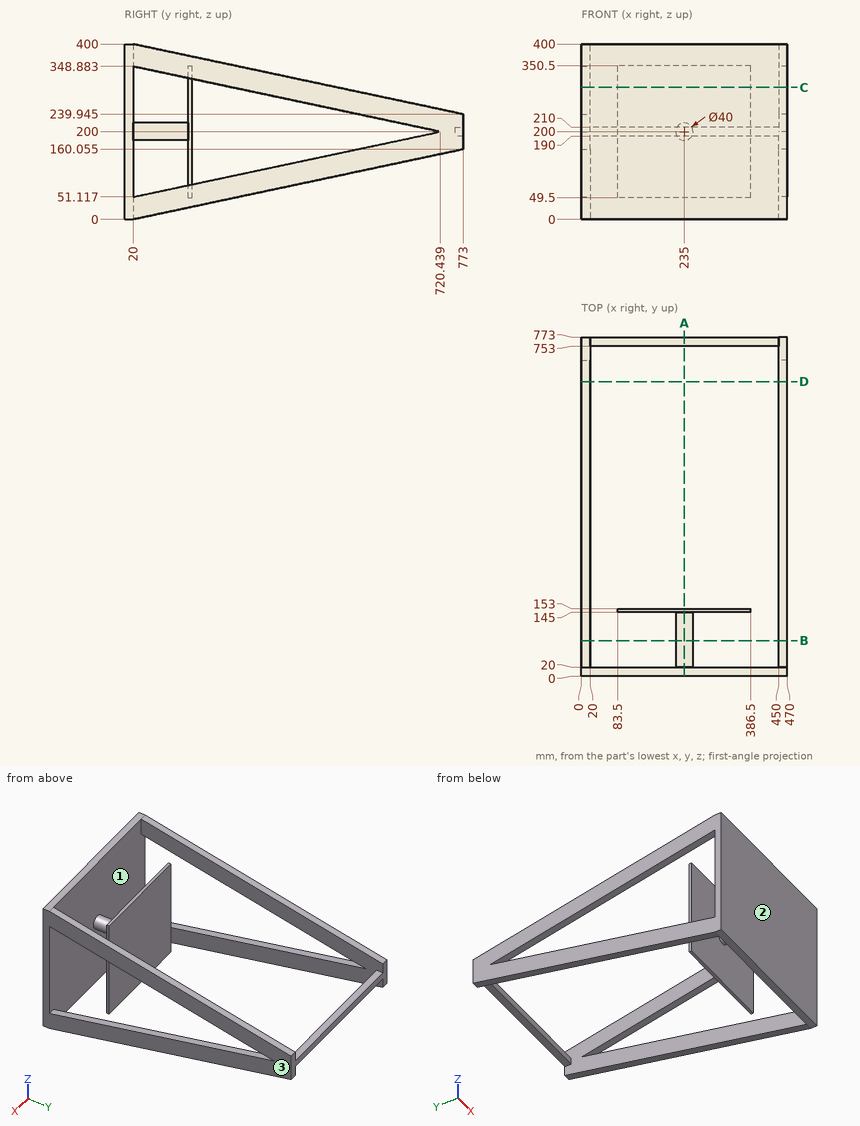
Can you work these out from the drawing? Everything is in mm from the part's minimum corner. Coordinates: 2 decimals unless noted, no trailing zeros. Loops run counter-clockwise (first coordinate to the right, second up) from the corner with the lowest first, then second, coordinate; pieces in that order, holes last. Notation, with made-up numbers: (-38.5, 72.5) - (-10.5, 72.5) arc R25 ccw to (-10.5, 94.5) - close; hole circle Ø9 at (0.5, 22). An arc over 180 degrees is marked (long way). Use a Markdown table: item, result.
Item 1: Will these pins go through, and if not, where does the flat tip stop? pin 1 (10 mm diameter, centred on x = 354.5, y = 146.5, fed in from +Z); pin 2 (22 mm diameter, centred on x = 159.5, y = 762.5, fed in from +Z); pin 3 (4 mm diameter, centred on y = 150, z = 266, fed in from -X).
Numbers:
| item | result |
|---|---|
| pin 1 | stops at z = 350.5 |
| pin 2 | stops at z = 210 |
| pin 3 | stops at x = 83.5 |
Item 2: We'd pull the mould along Y, two halves only. Please class the marked faces 1, 2 and 3: released by +Y, released by -Y, zero draft, split by the parting line, or undercut.
Numbers:
| item | result |
|---|---|
| face 1 | undercut |
| face 2 | released by -Y |
| face 3 | zero draft |
Item 3: I want a section at C-C on z = 301. Please give me the cut outline in (x, y).
Numbers:
| item | result |
|---|---|
| outline | (0, 0) - (470, 0) - (470, 20) - (0, 20) - close; (0, 245.27) - (20, 245.27) - (20, 485.76) - (0, 485.76) - close; (83.5, 145) - (386.5, 145) - (386.5, 153) - (83.5, 153) - close; (450, 245.27) - (470, 245.27) - (470, 485.76) - (450, 485.76) - close |
Item 4: I want a section at B-B on y = 81. Please give me the cut outline in (x, z), and give its area (3 significant figures).
Numbers:
| item | result |
|---|---|
| outline | (0, 12.97) - (20, 12.97) - (20, 64.08) - (0, 64.08) - close; (0, 335.92) - (20, 335.92) - (20, 387.03) - (0, 387.03) - close; circle Ø40 at (235, 200); (450, 12.97) - (470, 12.97) - (470, 64.08) - (450, 64.08) - close; (450, 335.92) - (470, 335.92) - (470, 387.03) - (450, 387.03) - close |
| area | 5,350 mm2 |
Item 5: I want a section at D-D on y = 672. Please give me the cut outline in (x, z), and give its area (3 significant figures).
Numbers:
| item | result |
|---|---|
| outline | (0, 138.59) - (20, 138.59) - (20, 189.7) - (0, 189.7) - close; (0, 210.3) - (20, 210.3) - (20, 261.41) - (0, 261.41) - close; (450, 138.59) - (470, 138.59) - (470, 189.7) - (450, 189.7) - close; (450, 210.3) - (470, 210.3) - (470, 261.41) - (450, 261.41) - close |
| area | 4,090 mm2 |
Item 6: If I drill on probe 1 along Y at (x, z) = (114, 202); probe 2 along Y at (x, z) = (189, 149); probe 3 along X at (y, z) = (402.5, 101.5), over which ranges is the centre line in solid material (lowest first)? Write a range as from..to.
Numbers:
| item | result |
|---|---|
| probe 1 | y = 0..20, 145..153, 753..773 |
| probe 2 | y = 0..20, 145..153 |
| probe 3 | x = 0..20, 450..470 |
Item 7: I want a section at A-A on x = 235. Please give me the cut outline in (y, z).
Numbers:
| item | result |
|---|---|
| outline | (0, 0) - (20, 0) - (20, 180) - (145, 180) - (145, 49.5) - (153, 49.5) - (153, 350.5) - (145, 350.5) - (145, 220) - (20, 220) - (20, 400) - (0, 400) - close; (753, 190) - (773, 190) - (773, 210) - (753, 210) - close |
